For this review, take the finished solid that the model builds, in its own axes (mm). Face numbers are marked on the shaded views. A direction names the side the tool comes from. Round coordinates to 2 decimals unless told otherwise and drop trailing zeros. Loops run counter-clockwise (first coordinate to the right, second up) from the corner with the lowest first, then second, coordinate; pieces in that order, holes last. Notation, with made-up numbers: (-27, 2) -> (12, 2) arc R20 cw to (12, 19) -> close; hole circle Ø5 at (17.5, 12.25). An arc over 180 degrees is marked (long way). One line per question, with ' | ' between items. Start each with the question number.
1. Consider section C-C (x = 14.5). Write out the cut boundary in (y, z).
2. Consider section B-B (x = -5). Write out the cut boundary in (y, z).
3. For pin 1 Ø3 at (y, z) = (-0.5, -1) entering from +X; pin 2 Ø1.4 at (x, z) = (14.5, -0.5) entering from -Y; pin 3 Ø1 at (x, y) = (7.5, 4.5) entering from +Z; pin 4 Ø2 at (x, y) = (-5.5, -5.5) entering from -Z, all flat-tipped, find the tip position at first contact; note any pin that passes through.
4. For the marked faces 1, 2, 3 and 4, list the 3-axis set-ups (+Z, -Z, +X, -X, +Y, -Y) from which the entire face can be reached by the end or side of a thin tool; tool diameter is ignored.
5. Wall thickness on line 1 along Y through (x, z) = (1.5, 0.25); line 2 along X through (y, z) = (-5.5, -2.25); line 3 along Y through (x, z) = (3, 0.5): over which ranges is each line inside the solid? List them lowest first.
6. Draft analysis for pull direction X (two halves, no side actions). For the marked faces 5, 6 and 7, state which applies: pulls with the +X half, pulls with the -X half, needs draft (parallel to the pull), parting line crosses it, or undercut.
```python
from build123d import *

# Parameters (mm, degrees)
F2_R     = 1
F4_DEPTH = 32
F5_DEPTH = 32
F6_DEPTH = 15
F7_DEPTH = 15
F8_DEPTH = 15
F9_R     = 0.2


with BuildPart() as f1:
    # F0 (on Front) → F1 (revolve)
    with BuildSketch(Plane.XZ):
        Polygon((-9.0454753935, 5.269), (-9.0454753935, 3.769), (22.9545246065, 3.769), (22.9545246065, 4.769), (18.9545246065, 4.769), (18.9545246065, 5.269), (11.4545246065, 5.269), (10.9545246065, 5.569), (10.4545246065, 5.269), (7.9545246065, 5.269), (7.9545246065, 7.269), (5.9545246065, 7.269), (5.9545246065, 5.269), align=None)
    revolve(axis=Axis((2.1683473801, 0, 0), (1, 0, 0)))

    # F2
    f2_edges = [f1.edges().sort_by_distance(p)[0] for p in [
        (5.954525, 0, -7.269),
    ]]
    fillet(f2_edges, radius=F2_R)

    # F3 (on face) → F4 (join)
    with BuildSketch(Plane(origin=(-9.0454753935, 0, 0), x_dir=(0, -1, 0), z_dir=(-1, 0, 0))):
        with BuildLine():
            ThreePointArc((3.769, 0), (3.6405744393, 0.975488981), (3.2640497469, 1.8845))
            Line((3.2640497469, 1.8845), (3.2640497469, -1.8845))
            ThreePointArc((3.2640497469, -1.8845), (3.6405744393, -0.975488981), (3.769, 0))
        make_face()
    extrude(amount=-F4_DEPTH)

    # F3 (on face) → F5 (join)
    with BuildSketch(Plane(origin=(-9.0454753935, 0, 0), x_dir=(0, -1, 0), z_dir=(-1, 0, 0))):
        with BuildLine():
            ThreePointArc((3.769, 0), (3.6405744393, 0.975488981), (3.2640497469, 1.8845))
            Line((3.2640497469, 1.8845), (3.2640497469, -1.8845))
            ThreePointArc((3.2640497469, -1.8845), (3.6405744393, -0.975488981), (3.769, 0))
        make_face()
        with BuildLine():
            Line((2.7877357748, 2.1595), (3.2640497469, 1.8845))
            ThreePointArc((3.2640497469, 1.8845), (3.1012168176, 2.1419185909), (2.9181290377, 2.3853477564))
            Line((2.9181290377, 2.3853477564), (2.7877357748, 2.1595))
        make_face()
        with BuildLine():
            ThreePointArc((1.0163546733, -3.6293779327), (2.3111934688, -2.9772043514), (3.2640497469, -1.8845))
            Line((3.2640497469, -1.8845), (0.8227241336, -3.294))
            Line((0.8227241336, -3.294), (1.0163546733, -3.6293779327))
        make_face()
        with BuildLine():
            Line((0, 3.769), (2.4413256133, 2.3595))
            Line((2.4413256133, 2.3595), (2.634956153, 2.6948779327))
            ThreePointArc((2.634956153, 2.6948779327), (1.4227378662, 3.4901544327), (0, 3.769))
        make_face()
        with BuildLine():
            Line((0.606707235, -3.7198477564), (0.4763139721, -3.494))
            Line((0.4763139721, -3.494), (0, -3.769))
            ThreePointArc((0, -3.769), (0.3043475037, -3.7566918422), (0.606707235, -3.7198477564))
        make_face()
        with BuildLine():
            Line((-3.2640497469, 1.8845), (0, 3.769))
            ThreePointArc((0, 3.769), (-1.8845, 3.2640497469), (-3.2640497469, 1.8845))
        make_face()
        with BuildLine():
            ThreePointArc((-3.2640497469, -1.8845), (-1.8845, -3.2640497469), (0, -3.769))
            Line((0, -3.769), (-3.2640497469, -1.8845))
        make_face()
        with BuildLine():
            Line((-3.2640497469, 1.3345), (-3.2640497469, 1.8845))
            ThreePointArc((-3.2640497469, 1.8845), (-3.4055643214, 1.6147732513), (-3.5248362728, 1.3345))
            Line((-3.5248362728, 1.3345), (-3.2640497469, 1.3345))
        make_face()
        with BuildLine():
            ThreePointArc((-3.6513108263, 0.9345), (-3.7339313349, -0.5129500813), (-3.2640497469, -1.8845))
            Line((-3.2640497469, -1.8845), (-3.2640497469, 0.9345))
            Line((-3.2640497469, 0.9345), (-3.6513108263, 0.9345))
        make_face()
    extrude(amount=-F5_DEPTH)

    # F3 (on face) → F6 (cut)
    with BuildSketch(Plane(origin=(-9.0454753935, 0, 0), x_dir=(0, -1, 0), z_dir=(-1, 0, 0))):
        with BuildLine():
            ThreePointArc((2.634956153, 2.6948779327), (2.78085257, 2.5440558138), (2.9181290377, 2.3853477564))
            Line((2.9181290377, 2.3853477564), (3.704312025, 3.7470566344))
            ThreePointArc((3.704312025, 3.7470566344), (3.5558605867, 3.8882150774), (3.402034372, 4.0234963814))
            Line((3.402034372, 4.0234963814), (2.634956153, 2.6948779327))
        make_face()
    extrude(amount=-F6_DEPTH, mode=Mode.SUBTRACT)

    # F3 (on face) → F7 (cut)
    with BuildSketch(Plane(origin=(-9.0454753935, 0, 0), x_dir=(0, -1, 0), z_dir=(-1, 0, 0))):
        with BuildLine():
            Line((1.7834328924, -4.9579963814), (1.0163546733, -3.6293779327))
            ThreePointArc((1.0163546733, -3.6293779327), (0.8127906784, -3.6803168767), (0.606707235, -3.7198477564))
            Line((0.606707235, -3.7198477564), (1.3928902223, -5.0815566344))
            ThreePointArc((1.3928902223, -5.0815566344), (1.589362739, -5.0235731391), (1.7834328924, -4.9579963814))
        make_face()
    extrude(amount=-F7_DEPTH, mode=Mode.SUBTRACT)

    # F3 (on face) → F8 (cut)
    with BuildSketch(Plane(origin=(-9.0454753935, 0, 0), x_dir=(0, -1, 0), z_dir=(-1, 0, 0))):
        with BuildLine():
            Line((-3.5248362728, 1.3345), (-5.0972022473, 1.3345))
            ThreePointArc((-5.0972022473, 1.3345), (-5.1452233257, 1.1353580617), (-5.1854672644, 0.9345))
            Line((-5.1854672644, 0.9345), (-3.6513108263, 0.9345))
            ThreePointArc((-3.6513108263, 0.9345), (-3.5936432484, 1.1362610629), (-3.5248362728, 1.3345))
        make_face()
    extrude(amount=-F8_DEPTH, mode=Mode.SUBTRACT)

    # F9
    f9_edges = [f1.edges().sort_by_distance(p)[0] for p in [
        (-9.045475, 1.589363, 5.023573),
        (-9.045475, -5.145223, -1.135358),
        (-9.045475, 3.555861, -3.888215),
        (-9.045475, 3.26405, -0.475),
        (-9.045475, 1.632025, -2.82675),
        (-9.045475, -0.238157, -3.6315),
        (-9.045475, -3.26405, 0),
        (-9.045475, -3.025893, 2.022),
        (-9.045475, 1.632025, 2.82675),
        (-9.045475, -1.220663, 3.06425),
        (-9.045475, -2.043387, -2.58925),
        (-9.045475, 3.26405, 1.6095),
    ]]
    fillet(f9_edges, radius=F9_R)


solid = f1.part
```
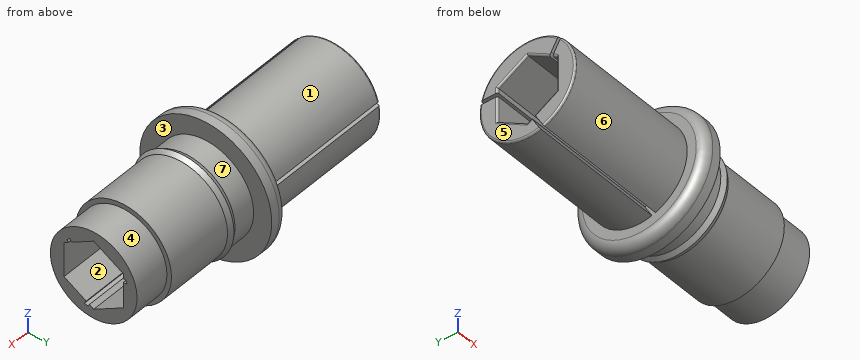
Answer block:
1) outline: circle Ø10.54 at (0, 0); hole (-3.26, -1.88) -> (-0.82, -3.29) -> (-1.02, -3.63) arc R3.77 ccw to (-0.61, -3.72) -> (-0.48, -3.49) -> (0, -3.77) -> (3.26, -1.88) -> (3.26, 0.93) -> (3.65, 0.93) arc R3.77 ccw to (3.52, 1.33) -> (3.26, 1.33) -> (3.26, 1.88) -> (0, 3.77) -> (-2.44, 2.36) -> (-2.63, 2.69) arc R3.77 ccw to (-2.92, 2.39) -> (-2.79, 2.16) -> (-3.26, 1.88) -> close
2) outline: (-3.7, 3.75) arc R5.27 ccw to (-1.78, -4.96) -> (-0.82, -3.29) -> (-3.26, -1.88) -> (-3.26, 1.88) -> (-2.79, 2.16) -> close; (-3.4, 4.02) -> (-2.44, 2.36) -> (0, 3.77) -> (3.26, 1.88) -> (3.26, 1.33) -> (5.1, 1.33) arc R5.27 ccw to start; (-1.39, -5.08) arc R5.27 ccw to (5.19, 0.93) -> (3.26, 0.93) -> (3.26, -1.88) -> (0, -3.77) -> (-0.48, -3.49) -> close
3) pin 1: passes through | pin 2: stops at y = -5.27 | pin 3: stops at z = 6.07 | pin 4: stops at z = -2.74
4) face 1: +Z, -X | face 2: +X, -X | face 3: none | face 4: +X
5) line 1: y = -5.26 to -3.26, 3.26 to 5.26 | line 2: x = 5.95 to 7.95 | line 3: y = -5.25 to -3.26, 3.26 to 5.25
6) face 5: pulls with the -X half | face 6: needs draft | face 7: undercut
